```python
from build123d import *

# Parameters (mm, degrees)
SKETCH_2_R          = 14
SKETCH_1_R          = 10.5
SKETCH_3_R          = 6.5
CUT_EXTRUDE_1_DEPTH = 10
SKETCH_4_R          = 2
CUT_EXTRUDE_2_DEPTH = 23.181073184


with BuildPart() as part:
    # Эскиз2 → По сечениям1 section 0
    with BuildSketch(Plane(origin=(0, 13, 0), x_dir=(1, 0, 0), z_dir=(0, 1, 0))):
        Circle(SKETCH_2_R)
    # Эскиз1 → По сечениям1 section 1
    with BuildSketch(Plane(origin=(0, 0, 0), x_dir=(1, 0, 0), z_dir=(0, 1, 0))):
        Circle(SKETCH_1_R)
    loft()

    # Эскиз3 → Вырез-Вытянуть1 (cut)
    with BuildSketch(Plane.XZ):
        with Locations(Location((0, 0, 0), (0, 0, 270))):
            Circle(SKETCH_3_R)
    extrude(amount=-CUT_EXTRUDE_1_DEPTH, mode=Mode.SUBTRACT)

    # Эскиз4 → Вырез-Вытянуть2 (cut, through all)
    with BuildSketch(Plane.XZ.offset(-10)):
        with Locations(Location((0, 0, 0), (0, 0, 270))):
            Circle(SKETCH_4_R)
    extrude(amount=-CUT_EXTRUDE_2_DEPTH, mode=Mode.SUBTRACT)


solid = part.part
```
Check sheet for the modelled part. Datum: model origin and axes. Units: mm. A direction names the side the tool comes from. Give positions to 0.01 mm unless a question says otherwise; leave off trailing zeros. Write each loop counter-clockwise with the first axis right and the second up, starting at its lowest first coordinate (ties: lowest second). Pieces come first, ordered by that corner, then holes. Notation, with made-up numbers: (28, 18.25) - (75, 18.25) arc R22 ccw to (75, 53.25) - close; hole circle Ø6 at (0, -30). An arc over 180 degrees is marked (long way). Answer as a JSON object with one key per item and string values. Group by question number.
1) Sectioned sample at B-B (y = 2.5). Record the cut outline in (x, z).
2) Access from +Z, -Z, +X, -X, +Y, -Y to the whole of each face (thin tool, end or side, straight path). Record for faces 5 (the face through (0, 13, 3)), 6 (the face through (-3.955, 4.93, 5.158)).
3) Depth check by flat-ended pin: P1, Ø5, axis at x = -2.5, y = 1.5, coming from the +Z side; P2, Ø3, axis at x = -6.5, y = 10.5, coming from the +Z side; P3, Ø3, axis at y = 9, z = -1, coming from the -X side. Enter the tip coordinate at first touch or a pass-through.
4) Release check for a two-part mould opening along Z. For faces 1 (the face through (2, 10, -1)), 2 (the face through (5, 0, -5)), 3 (the face through (-1.49, 3.52, -11.35)), 4 (the face through (-2, 11, 0)) record: pulls with the +Z half, pulls with the -Z half, needs draft (parallel to the pull), parting line crosses it, or undercut.
5) Sectioned sample at C-C (y = 1). Record the cut outline in (x, z), then the cut area to 3 significant figures.
6) Thickness scan on probe 1 along Z at (x, y) = (2.5, 8.5); probe 2 along X at (y, z) = (4.25, -0.75); probe 3 along X at (y, z) = (8, 5). Record the ranges inside material, lowest first. Write a range as from..to.
7) Sectioned sample at A-A (x = 0). Record the cut outline in (y, z), then the cut area to 4 significant figures.
Geometry results:
{
 "1": {"outline": "circle Ø22.35 at (0, 0); hole circle Ø13 at (0, 0)"},
 "2": {"face 5": "+Z, -Z, +X, -X, +Y", "face 6": "-Y"},
 "3": {"P1": "stops at z = 11.42", "P2": "stops at z = 12.49", "P3": "stops at x = -13.3"},
 "4": {"face 1": "undercut", "face 2": "needs draft", "face 3": "parting line crosses it", "face 4": "undercut"},
 "5": {"outline": "circle Ø21.54 at (0, 0); hole circle Ø13 at (0, 0)", "area": "232 mm^2"},
 "6": {"probe 1": "z = -12.54..-6, 6..12.54", "probe 2": "x = -11.62..-6.46, 6.46..11.62", "probe 3": "x = -11.62..-4.15, 4.15..11.62"},
 "7": {"outline": "(0, -10.5) - (13, -14) - (13, -2) - (10, -2) - (10, -6.5) - (0, -6.5) - close; (0, 6.5) - (10, 6.5) - (10, 2) - (13, 2) - (13, 14) - (0, 10.5) - close", "area": "176.5 mm^2"}
}
